Could you check a few things on this model? Use its own coordinates, in mm. Coordinates: 2 decimals unless noted, no trailing zeros. Loops run counter-clockwise (first coordinate to the right, second up) from the corner with the lowest first, then second, coordinate; pieces in that order, holes last.
from build123d import *

# Parameters (mm, degrees)
F0_R     = 38.1
F0_R_2   = 31.75
F1_DEPTH = 123.825
F2_R     = 38.1
F3_DEPTH = 6.35
F4_R     = 5.08


# Not quite as in the source:
# - a fillet or chamfer that OpenCascade refuses, or shapes differently, is made with other operations: its cross-section is extruded or revolved along the edge and cut away or added


with BuildPart() as f1:
    # F0 (on Front) → F1 (new body)
    with BuildSketch(Plane.XZ):
        Circle(F0_R)
        Circle(F0_R_2, mode=Mode.SUBTRACT)
    extrude(amount=F1_DEPTH)

    # F2 (on Front) → F3 (join)
    with BuildSketch(Plane.XZ):
        Circle(F2_R)
    extrude(amount=F3_DEPTH)

    # F4
    f4_edges = [f1.edges().sort_by_distance(p)[0] for p in [
        (-31.75, -123.825, 0),
    ]]
    fillet(f4_edges, radius=F4_R)

    # F5: fillet of radius 5.08 on 1 edges, made by hand

    # F5_s1 → F5_t2 (revolve, cut)
    with BuildSketch(Plane.XY):
        with BuildLine():
            ThreePointArc((36.83, -123.825), (37.7719048812, -122.2609470592), (38.1, -120.4648958349))
            Line((38.1, -120.4648958349), (38.1, -123.825))
            Line((38.1, -123.825), (36.83, -123.825))
        make_face()
    revolve(axis=Axis((0, -123.825, 0), (0, -1, 0)), mode=Mode.SUBTRACT)


solid = f1.part
(1) Imagine slicing it at A-A, the plane z = 0. Write out the boundary of the cut face in (x, y) (3 decimals).
Answers:
outline: (-38.1, -120.465) arc R5.08 ccw to (-36.83, -123.825) arc R5.08 ccw to (-31.75, -118.745) - (-31.75, -6.35) - (31.75, -6.35) - (31.75, -118.745) arc R5.08 ccw to (36.83, -123.825) arc R5.08 ccw to (38.1, -120.465) - (38.1, 0) - (-38.1, 0) - close
(2) Imagine slicing it at B-B, the plane x = 0. Write out the boundary of the cut face in (y, z) (3 decimals), and give its area (3 significant figures).
Answers:
outline: (-123.825, -36.83) arc R5.08 ccw to (-120.465, -38.1) - (0, -38.1) - (0, 38.1) - (-120.465, 38.1) arc R5.08 ccw to (-123.825, 36.83) arc R5.08 ccw to (-118.745, 31.75) - (-6.35, 31.75) - (-6.35, -31.75) - (-118.745, -31.75) arc R5.08 ccw to start
area: 1,960 mm2
(3) For pin 1 (12 mm diameter, centred on y = -78, z = -11.5, fed in from -X); pin 2 (10 mm diameter, centred on y = -89, z = -22.5, fed in from -X); pin 3 (8 mm diameter, centred on x = -30, y = -107, fed in from -Z), each with a flat end and sliding along its axis, tell me the tip position at first contact or that it passes through.
Answers:
pin 1: stops at x = -37.7
pin 2: stops at x = -33.84
pin 3: stops at z = -27.85
(4) Imagine slicing it at C-C, the plane y = -113.5. Write out the boundary of the cut face in (x, z).
Answers:
outline: circle Ø76.2 at (0, 0); hole circle Ø63.5 at (0, 0)
(5) We'd pull the mould along X, two halves only. Please class faces 1 (the face through (0, -6.35, 0)), 2 (the face through (-30.235, -59.389, -23.183)), 3 (the face through (-1, 0, 1)): +X half, -X half, draft (parallel to the pull), parting line (faces both ways), or undercut.
Answers:
face 1: undercut
face 2: parting line
face 3: draft
(6) I need wall thicknesses on probe 1 along Z at (x, y) = (0, -75); probe 2 along Y at (x, z) = (8.5, 27.5); probe 3 along Z at (x, y) = (9, -109). Which ranges of each line are inside material? Lowest first, please.
Answers:
probe 1: z = -38.1 to -31.75, 31.75 to 38.1
probe 2: y = -6.35 to 0
probe 3: z = -37.02 to -30.45, 30.45 to 37.02
